```python
from build123d import *

# Parameters (mm, degrees)
CHAMFER_1_SIZE = 2
CHAMFER_2_SIZE = 1


with BuildPart() as part:
    # Эскиз1 → Повернуть1 (revolve)
    with BuildSketch(Plane.XY, mode=Mode.PRIVATE) as revolve_1_sk:
        Polygon((-20, 30), (20, 30), (20, 14), (11, 14), (11, 12.5), (-11, 12.5), (-11, 14), (-20, 14), align=None)
    revolve(revolve_1_sk.sketch.rotate(Axis((0, 0, 0), (-1, 0, 0)), 90), axis=Axis((0, 0, 0), (-1, 0, 0)))

    # Фаска1
    chamfer_1_edges = [part.edges().sort_by_distance(p)[0] for p in [
        (-20, 0, 30),
        (20, 0, 30),
    ]]
    chamfer(chamfer_1_edges, length=CHAMFER_1_SIZE)

    # Фаска2
    chamfer_2_edges = [part.edges().sort_by_distance(p)[0] for p in [
        (-20, 0, 14),
        (20, 0, 14),
    ]]
    chamfer(chamfer_2_edges, length=CHAMFER_2_SIZE)


solid = part.part
```
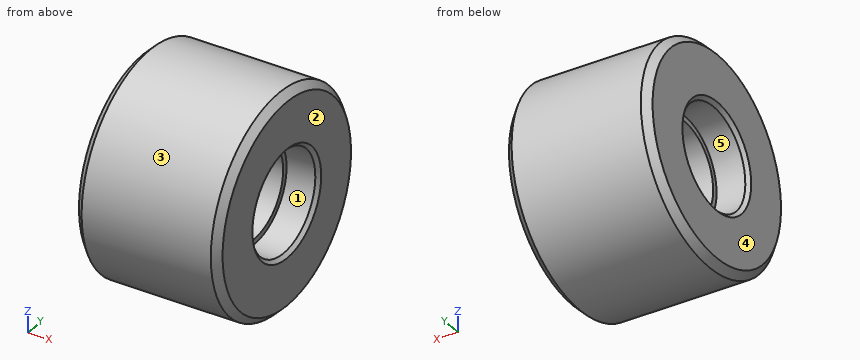
The listing builds one solid part. Answer for the finished solid, in the listing's coordinates (mm). Face numbers are marked on the shaded views. A direction names the side the tool comes from. Give positions to 0.01 mm unless a question says otherwise; leave off trailing zeros. Order: outer loops, then holes, each group sorted by start corner. A loop starts at its lowest first (then second) coordinate and runs counter-clockwise, first axis right, second up.
1) Consider line 1 along Y through (x, z) = (-16, 0); line 2 along Y through (x, z) = (4, 0); line 3 along Z through (x, y) = (-12.5, 11.5). Determine where each line is inside the solid, lowest interval first.
Reported:
line 1: y = -30 to -14, 14 to 30
line 2: y = -30 to -12.5, 12.5 to 30
line 3: z = -27.71 to -7.98, 7.98 to 27.71
2) For the marked faces 4 and 5, determine the directions among +Z, -Z, +X, -X, +Y, -Y from which every point of the face is accessible in a straight line to the end or side of a thin tool.
Reported:
face 4: +Z, -Z, -X, +Y, -Y
face 5: -X
3) Find section C-C on x = 8.5. Write down the section's boundary in (y, z).
Reported:
outline: circle Ø60 at (0, 0); hole circle Ø25 at (0, 0)
4) Determine the mould class of the marked faces 1, 2 and 3 for opening direction Z: pulls with the +Z half, pulls with the -Z half, needs draft (parallel to the pull), parting line crosses it, or undercut.
Reported:
face 1: undercut
face 2: needs draft
face 3: parting line crosses it
5) Given P1, Ø6, axis at x = 14, y = 18, coming from the +Z side; P2, Ø10, axis at x = -3, y = -14, coming from the -Z side; P3, Ø22.5, axis at y = 0, z = 0, coming from the -X side; P4, Ø10, axis at x = 7, y = -11.5, coming from the +Z side, each flat-ended and moving along its own axis, determine where each tip first touches the part or whether it passes through.
Reported:
P1: stops at z = 25.98
P2: stops at z = -28.62
P3: passes through
P4: stops at z = 29.29
6) Find section A-A on z = 0. Write down the section's boundary in (x, y), then the cut area to 3 significant figures.
Reported:
outline: (-20, -28) - (-18, -30) - (18, -30) - (20, -28) - (20, -15) - (19, -14) - (11, -14) - (11, -12.5) - (-11, -12.5) - (-11, -14) - (-19, -14) - (-20, -15) - close; (-20, 15) - (-19, 14) - (-11, 14) - (-11, 12.5) - (11, 12.5) - (11, 14) - (19, 14) - (20, 15) - (20, 28) - (18, 30) - (-18, 30) - (-20, 28) - close
area: 1,340 mm2
